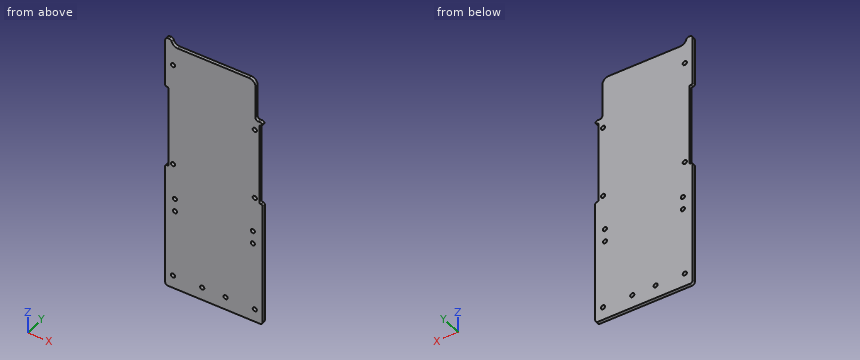
from build123d import *

# Parameters (mm, degrees)
SKETCH1_R               = 2.032
BOSS_EXTRUDE1_DEPTH     = 3.175
FILLET1_R               = 2.54
FILLET2_R               = 2.54
FILLET3_R               = 6.35
CUT_EXTRUDE1_DEPTH      = 136.673215063
FILLET4_R               = 6.35
FILLET5_R               = 2.54
SKETCH3_R               = 2.032
CUT_EXTRUDE2_DEPTH      = 136.673215063
CUT_EXTRUDE3_DEPTH      = 136.673215063
CUT_EXTRUDE3_DEPTH_BACK = 136.673215063
SKETCH4_W               = 3.175
SKETCH4_H               = 80.645
FILLET6_R               = 1.27


with BuildPart() as part:
    # Sketch1 → Boss-Extrude1 (new body)
    with BuildSketch(Plane(origin=(0, 0, 0), x_dir=(1, 0, 0), z_dir=(0, 1, 0))):
        Polygon((47.625, 127), (-47.625, 127), (-47.625, -127), (-41.275, -127), (-41.275, -120.65), (41.275, -120.65), (41.275, -127), (47.625, -127), align=None)
        with Locations(Location((-39.999684148, -101.6, 0), (0, 0, 270))):
            Circle(SKETCH1_R, mode=Mode.SUBTRACT)
        with Locations(Location((39.999684148, -69.85, 0), (0, 0, 270))):
            Circle(SKETCH1_R, mode=Mode.SUBTRACT)
        with Locations(Location((-39.999684148, 0, 0), (0, 0, 270))):
            Circle(SKETCH1_R, mode=Mode.SUBTRACT)
        with Locations(Location((-39.999684148, 114.3, 0), (0, 0, 270))):
            Circle(SKETCH1_R, mode=Mode.SUBTRACT)
        with Locations(Location((-11.424684148, 114.3, 0), (0, 0, 270))):
            Circle(SKETCH1_R, mode=Mode.SUBTRACT)
        with Locations(Location((39.999684148, 0, 0), (0, 0, 270))):
            Circle(SKETCH1_R, mode=Mode.SUBTRACT)
        with Locations(Location((11.424684148, 114.3, 0), (0, 0, 270))):
            Circle(SKETCH1_R, mode=Mode.SUBTRACT)
        with Locations(Location((39.999684148, 114.3, 0), (0, 0, 270))):
            Circle(SKETCH1_R, mode=Mode.SUBTRACT)
    extrude(amount=BOSS_EXTRUDE1_DEPTH)

    # Fillet1
    fillet1_edges = [part.edges().sort_by_distance(p)[0] for p in [
        (-47.625, 1.5875, 127),
        (-47.625, 1.5875, -127),
        (47.625, 1.5875, -127),
        (47.625, 1.5875, 127),
    ]]
    fillet(fillet1_edges, radius=FILLET1_R)

    # Fillet2
    fillet2_edges = [part.edges().sort_by_distance(p)[0] for p in [
        (-41.275, 1.5875, 127),
        (41.275, 1.5875, 127),
    ]]
    fillet(fillet2_edges, radius=FILLET2_R)

    # Fillet3
    fillet3_edges = [part.edges().sort_by_distance(p)[0] for p in [
        (41.275, 1.5875, 120.65),
        (-41.275, 1.5875, 120.65),
    ]]
    fillet(fillet3_edges, radius=FILLET3_R)

    # Sketch2 → Cut-Extrude1 (cut, through all)
    with BuildSketch(Plane.XZ):
        with BuildLine():
            Line((40.64508, 123.578690235), (40.64508, 79.88808))
            Line((40.64508, 79.88808), (47.625, 79.88808))
            Line((47.625, 79.88808), (47.625, 124.46))
            ThreePointArc((47.625, 124.46), (46.881051224, 126.256051224), (45.085, 127))
            Line((45.085, 127), (43.815, 127))
            ThreePointArc((43.815, 127), (42.297059666, 126.496530663), (41.380880287, 125.185714286))
            ThreePointArc((41.380880287, 125.185714286), (41.069166069, 124.356476684), (40.64508, 123.578690235))
        make_face()
    extrude(amount=-CUT_EXTRUDE1_DEPTH, mode=Mode.SUBTRACT)

    # Fillet4
    fillet4_edges = [part.edges().sort_by_distance(p)[0] for p in [
        (40.64508, 1.5875, 123.578690235),
    ]]
    fillet(fillet4_edges, radius=FILLET4_R)

    # Fillet5
    fillet5_edges = [part.edges().sort_by_distance(p)[0] for p in [
        (47.625, 1.5875, 79.88808),
        (40.64508, 1.5875, 79.88808),
    ]]
    fillet(fillet5_edges, radius=FILLET5_R)

    # Sketch3 → Cut-Extrude2 (cut, through all)
    with BuildSketch(Plane.XZ):
        with Locations(Location((-38.103460155, -34.913768806, 0), (0, 0, 270))):
            Circle(SKETCH3_R)
        with Locations(Location((-38.103460155, -47.490173279, 0), (0, 0, 270))):
            Circle(SKETCH3_R)
        with Locations(Location((38.103460155, -47.490173279, 0), (0, 0, 90))):
            Circle(SKETCH3_R)
        with Locations(Location((38.103460155, -34.913768806, 0), (0, 0, 90))):
            Circle(SKETCH3_R)
    extrude(amount=-CUT_EXTRUDE2_DEPTH, mode=Mode.SUBTRACT)

    # Sketch4 → Cut-Extrude3 (cut, two sides: drawn at the far end of the back side and taken through both)
    with BuildSketch(Plane(origin=(0, 3.175, 0), x_dir=(1, 0, 0), z_dir=(0, 1, 0)).offset(-CUT_EXTRUDE3_DEPTH_BACK)):
        with Locations((-46.0375, -36.5125)):
            Rectangle(SKETCH4_W, SKETCH4_H)
        with Locations((46.0375, -36.5125)):
            Rectangle(SKETCH4_W, SKETCH4_H)
    extrude(amount=CUT_EXTRUDE3_DEPTH + CUT_EXTRUDE3_DEPTH_BACK, mode=Mode.SUBTRACT)

    # Fillet6
    fillet6_edges = [part.edges().sort_by_distance(p)[0] for p in [
        (-44.45, 1.5875, -3.81),
        (-47.625, 1.5875, -3.81),
        (-47.625, 1.5875, 76.835),
        (-44.45, 1.5875, 76.835),
        (44.45, 1.5875, 76.835),
        (47.625, 1.5875, 76.835),
        (44.45, 1.5875, -3.81),
        (47.625, 1.5875, -3.81),
    ]]
    fillet(fillet6_edges, radius=FILLET6_R)


solid = part.part
Model file for the job. Use its own axes, mm. Give positions to 0.01 mm unless a question says otherwise; leave off trailing zeros. Loops run counter-clockwise (first coordinate to the right, second up) from the corner with the lowest first, then second, coordinate; pieces in that order, holes last. Notation, with made-up numbers: (41, -1) - (52, -1) arc R9 cw to (52, 4) - close; hole circle Ø4 at (-28, 3). An arc over 180 degrees is marked (long way). Use one line per item in the form item = value.
(1) Drop flat-ended pins along their axis: P1, Ø3.5, axis at x = 40, z = 69.85, coming from the +Y side; P2, Ø0.7, axis at x = -46, y = 1.5, coming from the +Z side. Give the stop position or say it passes through.
Determined:
P1 = through
P2 = 126.94
(2) Cut at C-C (y = 2.4). Count the separate pieces of the cut face and the enclosed holes in it, then the cut area to 3 significant figures.
Determined:
separate_pieces = 1
enclosed_holes = 12
area = 22,700 mm^2
(3) Cut at B-B (z = 86.5). Give the cut face in (x, y) (3 decimals), then the cut area to 3 significant figures.
Determined:
outline = (-47.625, 0) - (40.645, 0) - (40.645, 3.175) - (-47.625, 3.175) - close
area = 280 mm^2
(4) Cut at A-A (x = 22). Give the cut face in (y, z) (3 decimals), then the cut area to 3 significant figures.
Determined:
outline = (0, -127) - (3.175, -127) - (3.175, 120.65) - (0, 120.65) - close
area = 786 mm^2
(5) Drill centre lines: L1, parallel to X at y = 0.85, z = 0; L2, parallel to Z at x = -41, y = 1.6; L3, parallel to X at y = 0.65, z = -36.5 (3 decimals). Where is each one in solid material? Low to high.
Determined:
L1 = -44.45 to -42.03, -37.97 to 37.97, 42.03 to 44.45
L2 = -127 to -116.07, -112.53 to -1.77, 1.77 to 99.83, 103.37 to 124.21
L3 = -47.625 to -39.373, -36.833 to 36.833, 39.373 to 47.625
